```python
from build123d import *

# Parameters (mm, degrees)
SZKIC1_W                    = 170
SZKIC1_H                    = 20
DODANIE_WYCI_GNI_CIE1_DEPTH = 5
GNIAZDO1_START              = 3
GNIAZDO1_OUTLINE_W          = 100
GNIAZDO1_OUTLINE_H          = 10
GNIAZDO1_DEPTH              = 1
GNIAZDO1_START_2            = 4
GNIAZDO1_2_OUTLINE_W        = 100
GNIAZDO1_2_OUTLINE_H        = 1
GNIAZDO1_2_DEPTH            = 1
SZKIC2_W                    = 100
SZKIC2_H                    = 10
WYTNIJ_WYCI_GNI_CIE1_DEPTH  = 10
SZKIC3_W                    = 2
SZKIC3_H                    = 10
WYTNIJ_WYCI_GNI_CIE2_DEPTH  = 2
SZKIC4_W                    = 2
SZKIC4_H                    = 10
WYTNIJ_WYCI_GNI_CIE3_DEPTH  = 2
SZKIC5_W                    = 104
SZKIC5_H                    = 2
WYTNIJ_WYCI_GNI_CIE4_DEPTH  = 1
SZKIC6_R                    = 1.7
WYTNIJ_WYCI_GNI_CIE5_DEPTH  = 10
WYTNIJ_WYCI_GNI_CIE6_DEPTH  = 5
SZKIC8_W                    = 38
SZKIC8_H                    = 6
WYTNIJ_WYCI_GNI_CIE7_DEPTH  = 10


# Read off the part's stored shape, not the designer's step: Gniazdo1
with BuildPart() as part:
    # Szkic1 → Dodanie-wyciągnięcie1 (new body)
    with BuildSketch(Plane.XY):
        with Locations((-52.199192033, 33.239845261)):
            Rectangle(SZKIC1_W, SZKIC1_H)
    extrude(amount=DODANIE_WYCI_GNI_CIE1_DEPTH)

    # Gniazdo1 outline → Gniazdo1 (cut)
    with BuildSketch(Plane.XY.offset(GNIAZDO1_START)):
        with Locations((-52.199192033, 28.239845261)):
            Rectangle(GNIAZDO1_OUTLINE_W, GNIAZDO1_OUTLINE_H)
    extrude(amount=GNIAZDO1_DEPTH, mode=Mode.SUBTRACT)

    # Gniazdo1 2 outline → Gniazdo1 2 (cut)
    with BuildSketch(Plane.XY.offset(GNIAZDO1_START_2)):
        with Locations((-52.199192033, 32.739845261)):
            Rectangle(GNIAZDO1_2_OUTLINE_W, GNIAZDO1_2_OUTLINE_H)
    extrude(amount=GNIAZDO1_2_DEPTH, mode=Mode.SUBTRACT)

    # Szkic2 → Wytnij-wyciągnięcie1 (cut)
    with BuildSketch(Plane.XY.offset(3)):
        with Locations((-52.199192033, 28.239845261)):
            Rectangle(SZKIC2_W, SZKIC2_H)
    extrude(amount=WYTNIJ_WYCI_GNI_CIE1_DEPTH, mode=Mode.SUBTRACT)

    # Szkic3 → Wytnij-wyciągnięcie2 (cut)
    with BuildSketch(Plane(origin=(-102.199192033, 0, 0), x_dir=(0, 0, -1), z_dir=(1, 0, 0))):
        with Locations((-4, 28.239845261)):
            Rectangle(SZKIC3_W, SZKIC3_H)
    extrude(amount=-WYTNIJ_WYCI_GNI_CIE2_DEPTH, mode=Mode.SUBTRACT)

    # Szkic4 → Wytnij-wyciągnięcie3 (cut)
    with BuildSketch(Plane.ZY.offset(2.199192033)):
        with Locations((4, 28.239845261)):
            Rectangle(SZKIC4_W, SZKIC4_H)
    extrude(amount=-WYTNIJ_WYCI_GNI_CIE3_DEPTH, mode=Mode.SUBTRACT)

    # Szkic5 → Wytnij-wyciągnięcie4 (cut)
    with BuildSketch(Plane.XZ.offset(-33.239845261)):
        with Locations((-52.199192033, 4)):
            Rectangle(SZKIC5_W, SZKIC5_H)
    extrude(amount=-WYTNIJ_WYCI_GNI_CIE4_DEPTH, mode=Mode.SUBTRACT)

    # Szkic6 → Wytnij-wyciągnięcie5 (cut)
    with BuildSketch(Plane(origin=(0, 0, 0), x_dir=(-1, 0, 0), z_dir=(0, 0, -1))):
        with Locations((72.199192033, 38.239845261)):
            Circle(SZKIC6_R)
        with Locations((32.199192033, 38.239845261)):
            Circle(SZKIC6_R)
    extrude(amount=-WYTNIJ_WYCI_GNI_CIE5_DEPTH, mode=Mode.SUBTRACT)

    # Szkic7 → Wytnij-wyciągnięcie6 (cut)
    with BuildSketch(Plane.XZ.offset(-23.239845261)):
        Polygon((-0.199192033, 3), (-104.199192033, 3), (-104.199192033, 5), (-137.199192033, 5), (-137.199192033, 3), (-137.653937347, 3), (-137.653937347, 0), (-0.199192033, 0), (33.231073198, 0), (33.231073198, 3), (33.231073198, 5), (-0.199192033, 5), align=None)
    extrude(amount=-WYTNIJ_WYCI_GNI_CIE6_DEPTH, mode=Mode.SUBTRACT)

    # Szkic8 → Wytnij-wyciągnięcie7 (cut)
    with BuildSketch(Plane.XY.offset(3)):
        with Locations((-75.199192033, 31.239845261)):
            Rectangle(SZKIC8_W, SZKIC8_H)
        with Locations((-29.199192033, 31.239845261)):
            Rectangle(SZKIC8_W, SZKIC8_H)
    extrude(amount=-WYTNIJ_WYCI_GNI_CIE7_DEPTH, mode=Mode.SUBTRACT)


solid = part.part
```
Model file for the job. Use its own axes, mm. A direction names the side the tool comes from. Give positions to 0.01 mm unless a question says otherwise; leave off trailing zeros. Write each loop counter-clockwise with the first axis right and the second up, starting at its lowest first coordinate (ties: lowest second). Pieces come first, ordered by that corner, then holes. Notation, with made-up numbers: (-3, 61.25) -> (26, 61.25) arc R24 cw to (26, 94.25) -> close; hole circle Ø6 at (6, 1). An arc over 180 degrees is marked (long way). Use CSV: the item, a comma, the result in double quotes. Start each with the question number.
1) Drill centre lines: L1, parallel to X at y = 29.5, z = 1.7; L2, parallel to X at y = 38.25, z = 3.25; L3, parallel to X at y = 31.5, z = 3.7. Where is each one in solid material? Low to high.
2) Cut at C-C on x = -40. List the corners of the cut face in (y, z), plus the area to 3 significant figures.
3) Cut at A-A on y = 31. List the corners of the cut face in (x, z).
4) Pin check, flat tips, straight feed: P1, Ø5, axis at x = -5.5, y = 31, coming from the +Z side; P2, Ø2, axis at x = -72.2, y = 38.24, coming from the +Z side; P3, Ø2, axis at x = -14.5, z = 3, coming from the -Y side. Stop position of each tip, or through.
5) Two-plate mould, pull along Y, no slides. Class faces 1 (the cylindrical face through (-33.82, 38.75, 2.46)), 2 (the flat face through (-116, 28.24, 3)), 3 (the flat face through (32.801, 36, 2)): released by +Y, released by -Y, zero draft, split by the parting line, or undercut.
6) Tool access for faces 4 (the flat face through (-53, 43.24, 2)), 5 (the flat face through (-10.199, 31, 2)), 6 (the flat face through (-5, 31, 3)): list every direction of +Z, -Z, +X, -X, +Y, -Y with a clear straight run to the whole face (end or side of a thin tool).
7) Cut at B-B on z = 0.9. List the corners of the cut face in (x, y), plus the area to 3 significant figures.
Final values:
1,L1,"x = -137.2 to -94.2, -56.2 to -48.2, -10.2 to 32.8"
1,L2,"x = -137.2 to -73.9, -70.5 to -33.9, -30.5 to 32.8"
1,L3,"x = -137.2 to -104.2, -0.2 to 32.8"
2,outline,"(34.24, 0) -> (43.24, 0) -> (43.24, 5) -> (34.24, 5) -> close"
2,area,"45.0 mm2"
3,outline,"(-137.2, 0) -> (-94.2, 0) -> (-94.2, 3) -> (-104.2, 3) -> (-104.2, 5) -> (-137.2, 5) -> close; (-56.2, 0) -> (-48.2, 0) -> (-48.2, 3) -> (-56.2, 3) -> close; (-10.2, 0) -> (32.8, 0) -> (32.8, 5) -> (-0.2, 5) -> (-0.2, 3) -> (-10.2, 3) -> close"
4,P1,"stops at z = 3"
4,P2,"passes through"
4,P3,"stops at y = 34.24"
5,face 1,"undercut"
5,face 2,"released by -Y"
5,face 3,"zero draft"
6,face 4,"+Z, -Z, +X, -X, +Y"
6,face 5,"+Z, -Z, -Y"
6,face 6,"+Z, -Y"
7,outline,"(-137.2, 28.24) -> (-94.2, 28.24) -> (-94.2, 34.24) -> (-56.2, 34.24) -> (-56.2, 28.24) -> (-48.2, 28.24) -> (-48.2, 34.24) -> (-10.2, 34.24) -> (-10.2, 28.24) -> (32.8, 28.24) -> (32.8, 43.24) -> (-137.2, 43.24) -> close; hole circle Ø3.4 at (-72.2, 38.24); hole circle Ø3.4 at (-32.2, 38.24)"
7,area,"2,080 mm2"
